For this review, take the finished solid that the model builds, in its own axes (mm). A direction names the side the tool comes from. Give positions to 0.01 mm unless a question says otherwise; leave off trailing zeros.
from build123d import *

# Parameters (mm, degrees)
BOSS_EXTRUDE1_DEPTH          = 10
BOSS_EXTRUDE2_DEPTH          = 1
BOSS_EXTRUDE2_DEPTH_BACK     = 11
REVOLVE1_ANGLE               = 90
CUT_REVOLVE1_ANGLE           = 45
CUT_REVOLVE1_OTHER_WAY_ANGLE = 90
BOSS_EXTRUDE3_DEPTH          = 5
BOSS_EXTRUDE3_DEPTH_BACK     = 5
BOSS_EXTRUDE4_DEPTH          = 5
BOSS_EXTRUDE4_DEPTH_BACK     = 5
SKETCH19_R                   = 1
CUT_EXTRUDE3_DEPTH           = 10
SKETCH24_R                   = 1
CUT_EXTRUDE4_DEPTH           = 10
SKETCH21_R                   = 2.5
CUT_EXTRUDE2_DEPTH           = 10


with BuildPart() as part:
    # Sketch1 → Boss-Extrude1 (new body)
    with BuildSketch(Plane.XY):
        with BuildLine():
            Line((186.280110435, 212.216863761), (189.127439812, 0))
            Line((189.127439812, 0), (0, 0))
            Line((0, 0), (0, 125.576698411))
            add(Edge.make_bspline(
                [(0, 125.576698411), (10.557001905, 132.837635912), (17.098165485, 150.751131911), (30.538510921, 175.76338894), (49.352217031, 203.04075133), (76.867896029, 207.296992896), (91.097956951, 209.776295723)],
                knots=[0, 0, 0, 0, 0.275246051, 0.426571591, 0.655828837, 1, 1, 1, 1], degree=3))
            add(Edge.make_bspline(
                [(91.097956951, 209.776295723), (122.565116695, 215.374757588), (154.60100966, 210.515513687), (186.280110435, 212.216863761)],
                knots=[0, 0, 0, 0, 1, 1, 1, 1], degree=3))
        make_face()
    extrude(amount=BOSS_EXTRUDE1_DEPTH)

    # Sketch3 → Boss-Extrude2 (add, two sides)
    with BuildSketch(Plane.XY.offset(10)) as boss_extrude2_sk:
        with BuildLine():
            Line((40.691917073, 127.565231362), (173.80372619, 127.565231362))
            Line((173.80372619, 127.565231362), (173.80372619, 199.679337801))
            add(Edge.make_bspline(
                [(40.691917073, 127.565231362), (46.771290341, 134.933306827), (53.369134393, 161.704453989), (78.457507643, 191.212262771), (124.31750344, 201.038762955), (152.264868916, 199.362802741), (173.80372619, 199.679337801)],
                knots=[0, 0, 0, 0, 0.16561761, 0.500501685, 0.611599227, 1, 1, 1, 1], degree=3))
        make_face()
    extrude(amount=BOSS_EXTRUDE2_DEPTH)
    extrude(boss_extrude2_sk.sketch, amount=-BOSS_EXTRUDE2_DEPTH_BACK)

    # Sketch4 → Revolve1 (revolve)
    with BuildSketch(Plane.XY.offset(10)):
        with BuildLine():
            Line((18.099024499, 100.001165305), (43.413071111, 100.001165305))
            ThreePointArc((43.413071111, 100.001165305), (30.756047805, 112.658188611), (18.099024499, 100.001165305))
        make_face()
    revolve(axis=Axis((18.099024499, 100.001165305, 10), (1, 0, 0)), revolution_arc=REVOLVE1_ANGLE)

    # Sketch7 → Cut-Revolve1 (revolve, cut)
    with BuildSketch(Plane.XZ.offset(-100.001165305)):
        with BuildLine():
            Line((19.785436848, 10), (41.915940994, 10))
            ThreePointArc((41.915940994, 10), (30.850688921, 20.07738513), (19.785436848, 10))
        make_face()
    revolve(axis=Axis((19.785436848, 100.001165305, 10), (1, 0, 0)), revolution_arc=CUT_REVOLVE1_ANGLE, mode=Mode.SUBTRACT)

    # Sketch7 → Cut-Revolve1 other way (revolve, cut)
    with BuildSketch(Plane.XZ.offset(-100.001165305)):
        with BuildLine():
            Line((19.785436848, 10), (41.915940994, 10))
            ThreePointArc((41.915940994, 10), (30.850688921, 20.07738513), (19.785436848, 10))
        make_face()
    revolve(axis=Axis((19.785436848, 100.001165305, 10), (-1, 0, 0)), revolution_arc=CUT_REVOLVE1_OTHER_WAY_ANGLE, mode=Mode.SUBTRACT)

    # Sketch17 → Boss-Extrude3 (add, two sides)
    with BuildSketch(Plane(origin=(0, 40, 0), x_dir=(-1, 0, 0), z_dir=(0, -1, 0))) as boss_extrude3_sk:
        with BuildLine():
            Line((-188.57501815, 0), (-189.57501815, 0))
            ThreePointArc((-189.57501815, 0), (-192.762810227, -4.99036016), (-189.57501815, -9.98072032))
            Line((-189.57501815, -9.98072032), (-188.57501815, -9.98072032))
            Line((-188.57501815, -9.98072032), (-188.57501815, 0))
        make_face()
    extrude(amount=BOSS_EXTRUDE3_DEPTH)
    extrude(boss_extrude3_sk.sketch, amount=-BOSS_EXTRUDE3_DEPTH_BACK)

    # Sketch18 → Boss-Extrude4 (add, two sides)
    with BuildSketch(Plane(origin=(0, 160, 0), x_dir=(-1, 0, 0), z_dir=(0, -1, 0))) as boss_extrude4_sk:
        with BuildLine():
            Line((-186.972854644, -10), (-187.472854644, -10))
            ThreePointArc((-187.472854644, -10), (-190.720096746, -5), (-187.472854644, 0))
            Line((-187.472854644, 0), (-186.972854644, 0))
            Line((-186.972854644, 0), (-186.972854644, -10))
        make_face()
    extrude(amount=BOSS_EXTRUDE4_DEPTH)
    extrude(boss_extrude4_sk.sketch, amount=-BOSS_EXTRUDE4_DEPTH_BACK)

    # Sketch19 → Cut-Extrude3 (cut)
    with BuildSketch(Plane.XZ.offset(-155)):
        with Locations((188.57501815, 5)):
            Circle(SKETCH19_R)
    extrude(amount=-CUT_EXTRUDE3_DEPTH, mode=Mode.SUBTRACT)

    # Sketch24 → Cut-Extrude4 (cut)
    with BuildSketch(Plane.XZ.offset(-35)):
        with Locations((190.94512502, 4.99518008)):
            Circle(SKETCH24_R)
    extrude(amount=-CUT_EXTRUDE4_DEPTH, mode=Mode.SUBTRACT)

    # Sketch21 → Cut-Extrude2 (cut)
    with BuildSketch(Plane(origin=(0, 45, 0), x_dir=(1, 0, 0), z_dir=(0, 1, 0))):
        with Locations((187.262810227, -4.99036016)):
            Circle(SKETCH21_R)
    extrude(amount=-CUT_EXTRUDE2_DEPTH, mode=Mode.SUBTRACT)


solid = part.part
1) To check wall thickness, follow line 1 (Z direction, x = 61, y = 135); line 2 (X direction, y = 105.5, z = 13); line 3 (Z direction, x = 89, y = 30). State the ranges of each line that lie inside material, in increasing order.
Answer sheet:
line 1: z = -1 to 11
line 2: x = 19.76 to 22.47, 39.23 to 41.75
line 3: z = 0 to 10
2) Clearance check with flat-ended pins moving along their axes: pin 1 (1.3 mm diameter, centred on x = 190.5, z = 3, fed in from +Y); pin 2 (0.5 mm diameter, centred on y = 175.5, z = 10.5, fed in from +X); pin 3 (3 mm diameter, centred on x = 124, z = 10.5, fed in from +Y); pin 4 (4 mm diameter, centred on x = 50.5, z = 13.5, fed in from -Y). State where each tip first meets the part, or that it passes through.
Answer sheet:
pin 1: stops at y = 165
pin 2: stops at x = 173.8
pin 3: stops at y = 212.55
pin 4: passes through
3) Draft analysis for pull direction Y (two halves, no side actions). For faces 1 (the face through (184.765, 40.07, 4.88)), 2 (the face through (96, 85, 0)), 3 (the face through (28.8, 100.001, 20.1)), state which applies: +Y half, -Y half, draft (parallel to the pull), parting line (faces both ways), or undercut.
Answer sheet:
face 1: undercut
face 2: draft
face 3: -Y half
4) Tool access review of faces 4 (the face through (121, 165, 11)), 5 (the face through (190.72, 160.07, 5.09)): name each direction out of +Z, -Z, +X, -X, +Y, -Y from which nothing blocks a thin tool from reaching the whole face with its end or side.
Answer sheet:
face 4: +Z, +X, -X, +Y, -Y
face 5: +X, +Y
